Read the model definition and answer for the solid it produces. Units are mm, in the model's axes. Face numbers are marked on the shaded views. A direction names the side the tool comes from. Give positions to 0.01 mm unless a question says otherwise; leave off trailing zeros. Order: outer loops, then holes, each group sorted by start corner. A loop starts at its lowest first (then second) coordinate and runs counter-clockwise, first axis right, second up. Notation, with made-up numbers: (50.25, 79.5) -> (90.25, 79.5) arc R11 cw to (90.25, 95.5) -> close; hole circle Ø1 at (67.5, -4.5). An arc over 180 degrees is marked (long way). Answer as CSV lines item,"result". Start each with the question number.
1) Flat-ended cylindrical pins translate along their axes: pin 1 Ø12 at (x, y) = (14, 15.5) entering from +Z; pin 2 Ø8 at (x, z) = (-27, 47.5) entering from -Y; pin 3 Ø8.5 at (x, y) = (-23, 6.5) entering from -Z; pin 4 Ø12 at (x, z) = (-5, 14.5) entering from -Y. Find the tip coordinate at first contact, or state that the pin passes through.
2) For the marked faces 4, 5 and 6, determine the directions among +Z, -Z, +X, -X, +Y, -Y from which every point of the face is accessible in a straight line to the end or side of a thin tool.
3) Find section C-C (y = 14.5). State how many separate pieces and enclosed holes the cut face has, and give its area (3 significant figures).
4) Straight lines are drawn through the part: L1, parallel to X at y = 14.5, z = -1.5; L2, parallel to X at y = 8.5, z = 38.5; L3, parallel to Z at x = -28, y = 23.5. For each, find the intervals that lie inside material, in ascending order. Write a range as from..to.
5) The mould has two halves that part along Y. Classify the marked faces 1, 2 and 3: +Y half, -Y half, draft (parallel to the pull), parting line (faces both ways), or undercut.
6) Find section B-B (z = 20.5). Determine the outline of the cut face in (x, y).
7) Find section D-D (x = 26.5). Determine the outline of the cut face in (y, z), and give its area (3 significant figures).
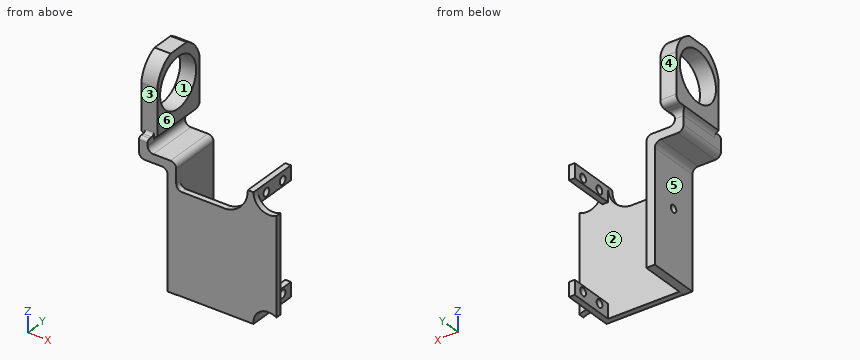
```python
from build123d import *

# Parameters (mm, degrees)
SKETCH1_W            = 31.75
SKETCH1_H            = 55.515999966
BOSS_EXTRUDE1_DEPTH  = 2.54
SKETCH10_W           = 8.89
SKETCH10_H           = 3.81
BOSS_EXTRUDE6_DEPTH  = 22.86
SKETCH12_W           = 7.112
SKETCH12_H           = 25.908
BOSS_EXTRUDE7_DEPTH  = 31.75
SKETCH13_R           = 11
SKETCH13_R_2         = 1.65
CUT_EXTRUDE5_DEPTH   = 21.59
SKETCH14_W           = 0.762
SKETCH14_H           = 14.055075912
CUT_EXTRUDE6_DEPTH   = 12.7
SKETCH15_W           = 2.54
SKETCH15_H           = 6.35
BOSS_EXTRUDE8_DEPTH  = 22.86
SKETCH16_R           = 1.750000056
CUT_EXTRUDE7_DEPTH   = 7.62
SKETCH17_W           = 42.815999966
SKETCH17_H           = 2.54
BOSS_EXTRUDE9_DEPTH  = 12.7
SKETCH18_W           = 5.08
SKETCH18_H           = 6.35
BOSS_EXTRUDE10_DEPTH = 2.54
CUT_EXTRUDE9_DEPTH   = 2.54
FILLET1_R            = 1.27
FILLET2_R            = 2.54
FILLET3_START        = 3.81
FILLET3_DEPTH        = 19.0499999
FILLET3_START_2      = 22.8599999
FILLET3_2_DEPTH      = 2.5400001
FILLET3_START_3      = -33
FILLET3_3_DEPTH      = 8.205718734


with BuildPart() as part:
    # Sketch1 → Boss-Extrude1 (new body)
    with BuildSketch(Plane(origin=(0, 0, 0), x_dir=(1, 0, 0), z_dir=(0, 1, 0))):
        with Locations((2.256707018, -2.686772311)):
            Rectangle(SKETCH1_W, SKETCH1_H)
    extrude(amount=BOSS_EXTRUDE1_DEPTH)

    # Sketch10 → Boss-Extrude6 (add)
    with BuildSketch(Plane(origin=(0, 0, 0), x_dir=(-1, 0, 0), z_dir=(0, -1, 0))):
        Polygon((13.618292982, 25.071227672), (13.618292982, -30.444772294), (17.428292982, -30.444772294), (17.428292982, -26.634772294), (17.428292982, 25.177062632), (13.618292982, 25.177062632), align=None)
        with Locations((21.873292982, -28.539772294)):
            Rectangle(SKETCH10_W, SKETCH10_H)
        Polygon((26.318292982, -26.634772294), (26.318292982, -30.444772294), (26.318292982, -35.526292066), (30.128292982, -35.526292066), (30.128292982, -26.634772294), align=None)
    extrude(amount=-BOSS_EXTRUDE6_DEPTH)

    # Sketch12 → Boss-Extrude7 (add)
    with BuildSketch(Plane.XY.offset(35.526292066)):
        with Locations((-28.350292982, 16.764)):
            Rectangle(SKETCH12_W, SKETCH12_H)
    extrude(amount=BOSS_EXTRUDE7_DEPTH)

    # Sketch13 → Cut-Extrude5 (cut)
    with BuildSketch(Plane.ZY.offset(31.906292982)):
        with BuildLine():
            Line((67.276292066, 3.81), (67.276292066, 14.316171348))
            ThreePointArc((67.276292066, 14.316171348), (63.220762226, 7.257694985), (55.846292066, 3.81))
            Line((55.846292066, 3.81), (67.276292066, 3.81))
        make_face()
        with BuildLine():
            ThreePointArc((55.846292066, 29.718), (63.159812447, 26.327226274), (67.276292066, 19.396171348))
            Line((67.276292066, 19.396171348), (67.276292066, 29.718))
            Line((67.276292066, 29.718), (55.846292066, 29.718))
        make_face()
        with Locations(Location((52.036292066, 16.51, 0), (0, 0, 270))):
            Circle(SKETCH13_R)
        with Locations((4.032937368, 11.43)):
            Circle(SKETCH13_R_2)
    extrude(amount=-CUT_EXTRUDE5_DEPTH, mode=Mode.SUBTRACT)

    # Sketch14 → Cut-Extrude6 (cut)
    with BuildSketch(Plane.ZY.offset(31.906292982)):
        with Locations((66.895292066, 16.391473574)):
            Rectangle(SKETCH14_W, SKETCH14_H)
    extrude(amount=-CUT_EXTRUDE6_DEPTH, mode=Mode.SUBTRACT)

    # Sketch15 → Boss-Extrude8 (add)
    with BuildSketch(Plane.XZ):
        with Locations((19.401707018, -21.896227672)):
            Rectangle(SKETCH15_W, SKETCH15_H)
        with Locations((19.401707018, 27.269772294)):
            Rectangle(SKETCH15_W, SKETCH15_H)
    extrude(amount=-BOSS_EXTRUDE8_DEPTH)

    # Sketch16 → Cut-Extrude7 (cut)
    with BuildSketch(Plane(origin=(20.671707018, 0, 0), x_dir=(0, 0, -1), z_dir=(1, 0, 0))):
        with Locations((-26.634772294, 7.874)):
            Circle(SKETCH16_R)
        with Locations((-26.634772294, 17.78)):
            Circle(SKETCH16_R)
        with Locations((21.261227672, 7.78)):
            Circle(SKETCH16_R)
        with Locations((21.261227672, 17.78)):
            Circle(SKETCH16_R)
    extrude(amount=-CUT_EXTRUDE7_DEPTH, mode=Mode.SUBTRACT)

    # Sketch17 → Boss-Extrude9 (add)
    with BuildSketch(Plane(origin=(18.131707018, 0, 0), x_dir=(0, 0, -1), z_dir=(1, 0, 0))):
        with Locations((-2.686772311, 1.27)):
            Rectangle(SKETCH17_W, SKETCH17_H)
    extrude(amount=BOSS_EXTRUDE9_DEPTH)

    # Sketch18 → Boss-Extrude10 (add)
    with BuildSketch(Plane(origin=(0, 2.54, 0), x_dir=(1, 0, 0), z_dir=(0, 1, 0))):
        with Locations((23.211707018, 21.896227672)):
            Rectangle(SKETCH18_W, SKETCH18_H)
        with Locations((23.211707018, -27.269772294)):
            Rectangle(SKETCH18_W, SKETCH18_H)
    extrude(amount=-BOSS_EXTRUDE10_DEPTH)

    # Sketch19 → Cut-Extrude9 (cut)
    with BuildSketch(Plane(origin=(0, 2.54, 0), x_dir=(1, 0, 0), z_dir=(0, 1, 0))):
        with BuildLine():
            Line((25.751707018, 25.071227672), (20.671707018, 25.071227672))
            Line((20.671707018, 25.071227672), (20.671707018, 24.618530893))
            Line((20.671707018, 24.618530893), (20.671707018, 24.032468758))
            ThreePointArc((20.671707018, 24.032468758), (21.560891333, 20.998252578), (23.754580952, 18.721227672))
            Line((23.754580952, 18.721227672), (25.751707018, 18.721227672))
            Line((25.751707018, 18.721227672), (25.751707018, 25.071227672))
        make_face()
        with BuildLine():
            Line((30.831707018, 18.721227672), (25.751707018, 18.721227672))
            Line((25.751707018, 18.721227672), (23.754580952, 18.721227672))
            ThreePointArc((23.754580952, 18.721227672), (27.293143985, 17.697581999), (30.831707018, 18.721227672))
        make_face()
        with BuildLine():
            ThreePointArc((18.131707018, -29.988694367), (15.379086377, -22.799421621), (8.675431219, -19.014772294))
            Line((8.675431219, -19.014772294), (-13.618292982, -19.014772294))
            Line((-13.618292982, -19.014772294), (-13.618292982, -30.444772294))
            Line((-13.618292982, -30.444772294), (18.131707018, -30.444772294))
            Line((18.131707018, -30.444772294), (18.131707018, -29.988694367))
        make_face()
        with BuildLine():
            Line((25.751707018, -24.094772294), (30.831707018, -24.094772294))
            ThreePointArc((30.831707018, -24.094772294), (24.069006733, -24.315202296), (20.671707018, -30.166788334))
            Line((20.671707018, -30.166788334), (20.671707018, -30.444772294))
            Line((20.671707018, -30.444772294), (25.751707018, -30.444772294))
            Line((25.751707018, -30.444772294), (25.751707018, -24.094772294))
        make_face()
    extrude(amount=-CUT_EXTRUDE9_DEPTH, mode=Mode.SUBTRACT)

    # Fillet1
    fillet1_edges = [part.edges().sort_by_distance(p)[0] for p in [
        (-28.223292982, 0, 35.526292066),
        (-28.223292982, 3.81, 35.526292066),
    ]]
    fillet(fillet1_edges, radius=FILLET1_R)

    # Fillet2
    fillet2_edges = [part.edges().sort_by_distance(p)[0] for p in [
        (-26.318292982, 11.43, 30.444772294),
        (-13.618292982, 11.43, 30.444772294),
        (-17.428292982, 11.43, 26.634772294),
        (-30.128292982, 11.43, 26.634772294),
        (-28.223292982, 22.86, 35.526292066),
        (-13.618292982, 1.27, 19.014772294),
        (-28.350292982, 29.718, 35.526292066),
    ]]
    fillet(fillet2_edges, radius=FILLET2_R)

    # Fillet3: read off the stored shape, not the designer's step
    # Fillet3 outline → Fillet3 (add)
    with BuildSketch(Plane(origin=(0, 0, 0), x_dir=(1, 0, 0), z_dir=(0, 1, 0)).offset(FILLET3_START)):
        with BuildLine():
            Line((-26.318292982, -35.526292066), (-24.794272712, -35.526300912))
            ThreePointArc((-24.794272712, -35.526300912), (-25.903403393, -34.589568161), (-26.318292982, -33.198343613))
            Line((-26.318292982, -33.198343613), (-26.318292982, -35.526292066))
        make_face()
        with BuildLine():
            Line((-31.906292982, -35.526292066), (-30.128292982, -35.526292066))
            Line((-30.128292982, -35.526292066), (-30.128292982, -33.103286494))
            ThreePointArc((-30.128292982, -33.103286494), (-30.620479514, -34.605970759), (-31.906292982, -35.526292066))
        make_face()
    extrude(amount=FILLET3_DEPTH)

    # Fillet3 2 outline → Fillet3 2 (add)
    with BuildSketch(Plane(origin=(0, 0, 0), x_dir=(1, 0, 0), z_dir=(0, 1, 0)).offset(FILLET3_START_2)):
        with BuildLine():
            Line((-26.318292982, -35.526292066), (-24.794272712, -35.526300912))
            ThreePointArc((-24.794272712, -35.526300912), (-25.903403393, -34.589568161), (-26.318292982, -33.198343613))
            Line((-26.318292982, -33.198343613), (-26.318292982, -35.526292066))
        make_face()
        with BuildLine():
            Line((-31.906292982, -35.526292066), (-30.128292982, -35.526292066))
            Line((-30.128292982, -35.526292066), (-30.128292982, -33.103286494))
            ThreePointArc((-30.128292982, -33.103286494), (-30.620479514, -34.605970759), (-31.906292982, -35.526292066))
        make_face()
    extrude(amount=FILLET3_2_DEPTH)

    # Fillet3 3 outline → Fillet3 3 (cut)
    with BuildSketch(Plane.YZ.offset(FILLET3_START_3)):
        with BuildLine():
            Line((25.4, 32), (25.4, 35.526292066))
            ThreePointArc((25.4, 35.526292066), (23.603948776, 34.78234329), (22.86, 32.986292066))
            Line((22.86, 32.986292066), (22.86, 32))
            Line((22.86, 32), (25.4, 32))
        make_face()
    extrude(amount=FILLET3_3_DEPTH, mode=Mode.SUBTRACT)


solid = part.part
```
Findings below:
1,pin 1,"z = 30.44"
1,pin 2,"y = 3.81"
1,pin 3,"z = 26.32"
1,pin 4,"y = 0"
2,face 4,"+Z, -Z, +X, -X, +Y"
2,face 5,"-Z, -X, +Y, -Y"
2,face 6,"+Z, +X, +Y, -Y"
3,separate pieces,"4"
3,enclosed holes,"0"
3,area,"381 mm²"
4,L1,"-17.43..-13.62"
4,L2,"-31.91..-24.79"
4,L3,"34.67..43.54, 60.53..65.54"
5,face 1,"undercut"
5,face 2,"+Y half"
5,face 3,"-Y half"
6,outline,"(-17.43, 0) -> (-13.39, 0) -> (-13.39, 2.54) -> (-13.62, 2.54) -> (-13.62, 22.86) -> (-17.43, 22.86) -> close; (12.66, 0) -> (30.83, 0) -> (30.83, 2.54) -> (12.66, 2.54) -> close"
7,outline,"(0, -17.75) -> (2.54, -17.75) -> (2.54, 23.42) -> (0, 23.42) -> close"
7,area,"105 mm²"
